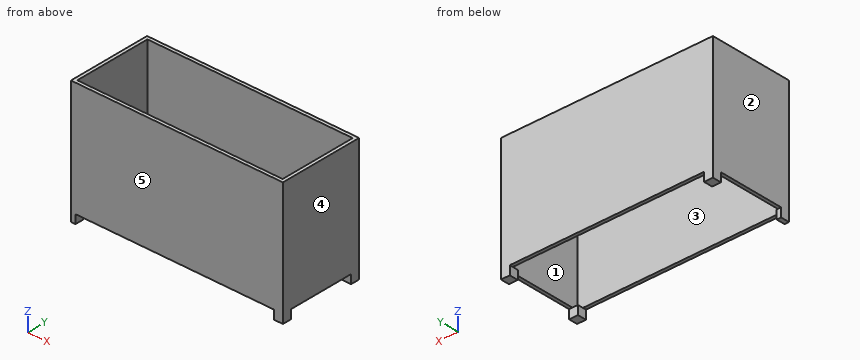
```python
from build123d import *

# Parameters (mm, degrees)
F0_W     = 1219.2
F0_H     = 711.2
F1_DEPTH = 482.6
F2_W     = 1117.6
F2_H     = 50.8
F3_DEPTH = 482.6
F4_W     = 381
F4_H     = 50.8
F5_DEPTH = 1219.2
F6_W     = 1181.1
F6_H     = 444.5
F7_DEPTH = 660.4
F8_W     = 25.4
F8_H     = 50.8
F9_DEPTH = 50.8


with BuildPart() as f1:
    # F0 (on Front) → F1 (new body)
    with BuildSketch(Plane.XZ):
        with Locations((19.749452, 355.6)):
            Rectangle(F0_W, F0_H)
    extrude(amount=-F1_DEPTH)

    # F2 (on face) → F3 (cut, through all)
    with BuildSketch(Plane.XZ):
        with Locations((19.749452, 25.4)):
            Rectangle(F2_W, F2_H)
    extrude(amount=-F3_DEPTH, mode=Mode.SUBTRACT)

    # F4 (on face) → F5 (cut, through all)
    with BuildSketch(Plane.YZ.offset(629.349452)):
        with Locations((241.3, 25.4)):
            Rectangle(F4_W, F4_H)
    extrude(amount=-F5_DEPTH, mode=Mode.SUBTRACT)

    # F6 (on face) → F7 (cut, through all)
    with BuildSketch(Plane.XY.offset(711.2)):
        with Locations((19.749452, 241.3)):
            Rectangle(F6_W, F6_H)
    extrude(amount=-F7_DEPTH, mode=Mode.SUBTRACT)

    # F8 (on face) → F9 (cut)
    with BuildSketch(Plane(origin=(0, 0, 0), x_dir=(1, 0, 0), z_dir=(0, 0, -1))):
        with Locations((-551.750548, -25.4)):
            Rectangle(F8_W, F8_H)
    extrude(amount=-F9_DEPTH, mode=Mode.SUBTRACT)


solid = f1.part
```
Geometry check sheet. Reference: the model listing, model coordinates, mm. Face numbers are marked on the shaded views. A direction names the side the tool comes from. Round coordinates to 2 decimals unless told otherwise and drop trailing zeros. Loops run counter-clockwise (first coordinate to the right, second up) from the corner with the lowest first, then second, coordinate; pieces in that order, holes last. Notation, with made-up numbers: M 83,6.5 L 135,6.5 A20 cw 135,15.5 Z; hole C -22,26 d7. An arc over 180 degrees is marked long. Return JSON: item names as keys, results as strings. Group by question number.
(1) Scan lines: line 1 along Y through (x, z) = (-147, 67); line 2 along X through (y, z) = (20.5, 682.5). Record each from-to range of solid material in increasing order. Write a range as [from, to].
(2) Mould release check, pull along X, two halves, no side actions. Record for the marked faces 3, 4 and 5: pulls with the +X half, pulls with the -X half, needs draft (parallel to the pull), parting line crosses it, or undercut.
(3) Section check A-A, the plane z = 353. Enter the section's corners in (x, y).
(4) Section check C-C, the plane y = 209. Enter the section's corners in (x, z).
(5) Section check B-B, the plane x = 122. Enter the section's corners in (y, z), and give its area (3 significant figures).
(6) Go/stop test with flat-tipped pins: pin 1 (9.5 mm diameter, centred on x = -556.5, y = 443, fed in from +Z); pin 2 (5 mm diameter, centred on x = -568.5, y = 30, fed in from +Z); pin 3 (9.5 mm diameter, centred on x = -244.5, y = 7, fed in from -Z). Record where each tip stops, or that it passes through.
(7) Set-up check for the marked faces 1 and 2: record each of +Z, -Z, +X, -X, +Y, -Y from which the full face is reachable in a straight line by a thin tool's end or side.
Data:
{
 "1": {"line 1": "[0, 19.05], [463.55, 482.6]", "line 2": "[-589.85, -570.8], [610.3, 629.35]"},
 "2": {"face 3": "undercut", "face 4": "pulls with the +X half", "face 5": "needs draft"},
 "3": {"outline": "M -589.85,0 L 629.35,0 L 629.35,482.6 L -589.85,482.6 Z; hole M -570.8,19.05 L 610.3,19.05 L 610.3,463.55 L -570.8,463.55 Z"},
 "4": {"outline": "M -589.85,50.8 L -570.8,50.8 L -570.8,711.2 L -589.85,711.2 Z; M 610.3,50.8 L 629.35,50.8 L 629.35,711.2 L 610.3,711.2 Z"},
 "5": {"outline": "M 0,50.8 L 19.05,50.8 L 19.05,711.2 L 0,711.2 Z; M 463.55,50.8 L 482.6,50.8 L 482.6,711.2 L 463.55,711.2 Z", "area": "25,200 mm²"},
 "6": {"pin 1": "z = 50.8", "pin 2": "z = 711.2", "pin 3": "z = 50.8"},
 "7": {"face 1": "+Z", "face 2": "+Z, -Z, -X, +Y, -Y"}
}
